```python
from build123d import *

# Parameters (mm, degrees)
SKETCH_1_R          = 25
EXTRUDE_1_DEPTH     = 15
SKETCH_2_R          = 11
CUT_EXTRUDE_1_DEPTH = 39.405728739
HOLE_WIZARD_M5_1_D  = 5.5


with BuildPart() as part:
    # ｽｹｯﾁ1 → ﾎﾞｽ - 押し出し1 (new body)
    with BuildSketch(Plane(origin=(0, 0, 0), x_dir=(1, 0, 0), z_dir=(0, 1, 0))):
        with Locations(Location((0, 0, 0), (0, 0, 270))):
            Circle(SKETCH_1_R)
    extrude(amount=EXTRUDE_1_DEPTH)

    # ｽｹｯﾁ2 → ｶｯﾄ - 押し出し1 (cut, through all)
    with BuildSketch(Plane(origin=(0, 15, 0), x_dir=(1, 0, 0), z_dir=(0, 1, 0))):
        with Locations(Location((0, 0, 0), (0, 0, 270))):
            Circle(SKETCH_2_R)
    extrude(amount=-CUT_EXTRUDE_1_DEPTH, mode=Mode.SUBTRACT)

    # M5 すきま穴1 (through all)
    with Locations(Plane(origin=(0, 15, 0), x_dir=(1, 0, 0), z_dir=(0, 1, 0))):
        with Locations((-12.727922061, 12.727922061), (12.727922061, -12.727922061), (-12.727922061, -12.727922061), (12.727922061, 12.727922061)):
            Hole(HOLE_WIZARD_M5_1_D / 2)


solid = part.part
```
Here's how the part is built. I have some questions about the finished solid (model axes, mm). Coordinates: 2 decimals unless noted, no trailing zeros. Order: outer loops, then holes, each group sorted by start corner. A loop starts at its lowest first (then second) coordinate and runs counter-clockwise, first axis right, second up.
Item 1: Thinking about a two-plate mould opening in Z: for faces 1 (the face through (-10.74, 7.6, -2.38)), 2 (the face through (-10.7, 7.39, 10.87)), 3 (the face through (-5, 0, 11)), 4 (the face through (7.509, 7.395, 23.846)), which applies, pulls with the +Z half, pulls with the -Z half, needs draft (parallel to the pull), parting line crosses it, or undercut?
Response values:
face 1: undercut
face 2: undercut
face 3: needs draft
face 4: parting line crosses it
Item 2: If we section it at A-A, the plane z = 0: List the corners of the cut face in (x, y) for me.
Response values:
outline: (-25, 0) - (-11, 0) - (-11, 15) - (-25, 15) - close; (11, 0) - (25, 0) - (25, 15) - (11, 15) - close
Item 3: I need wall thicknesses on probe 1 along X at (y, z) = (8.25, -14); probe 2 along X at (y, z) = (9, 13); probe 3 along Z at (x, y) = (15, 2). Which ranges of each line are inside material? Lowest first, please.
Response values:
probe 1: x = -20.71 to -15.17, -10.29 to 10.29, 15.17 to 20.71
probe 2: x = -21.35 to -15.46, -9.99 to 9.99, 15.46 to 21.35
probe 3: z = -20 to -14.28, -11.18 to 11.18, 14.28 to 20
Item 4: If we section it at D-D, the plane y = 11.5: List the corners of the cut face in (x, z) for me.
Response values:
outline: circle Ø50 at (0, 0); hole circle Ø5.5 at (-12.73, -12.73); hole circle Ø5.5 at (-12.73, 12.73); hole circle Ø22 at (0, 0); hole circle Ø5.5 at (12.73, -12.73); hole circle Ø5.5 at (12.73, 12.73)
Item 5: If we section it at B-B, the plane x = 0: List the corners of the cut face in (y, z) for me, then the cut area to 3 significant figures.
Response values:
outline: (0, -25) - (15, -25) - (15, -11) - (0, -11) - close; (0, 11) - (15, 11) - (15, 25) - (0, 25) - close
area: 420 mm2
Item 6: I'm going to push flat-ended pins straight in: pin 1 Ø20 at (x, z) = (0, 0) entering from -Y; pin 2 Ø5 at (y, z) = (11, 6.5) entering from -X; pin 3 Ø2 at (y, z) = (11.5, -3) entering from -X; pin 4 Ø1.5 at (x, y) = (-17.5, 3.5) entering from +Z. Where does each tip first touch, or does it pass through?
Response values:
pin 1: passes through
pin 2: stops at x = -24.68
pin 3: stops at x = -24.92
pin 4: stops at z = 18.56
Item 7: If we section it at C-C, the plane x = 14: List the corners of the cut face in (y, z) for me.
Response values:
outline: (0, -20.71) - (15, -20.71) - (15, -15.17) - (0, -15.17) - close; (0, -10.29) - (15, -10.29) - (15, 10.29) - (0, 10.29) - close; (0, 15.17) - (15, 15.17) - (15, 20.71) - (0, 20.71) - close
